Could you check a few things on this model? Use its own coordinates, in mm. A direction names the side the tool comes from. Coordinates: 2 decimals unless noted, no trailing zeros. Order: outer loops, then holes, each group sorted by start corner. A loop starts at its lowest first (then second) coordinate and runs counter-clockwise, first axis right, second up. Notation, with made-up numbers: (74, -20.5) - (85, -20.5) arc R18 ccw to (85, -9.5) - close; hole circle Ø6 at (38, 7.25). An arc over 180 degrees is marked (long way). One line per item, written item: value.
Autodesk Inventor part; units mm, degrees
ref_plane "Work Plane1" through (18.7433, 3, 13) normal (0, -1, 0) x (1, 0, 0)
ref_plane "YZ Plane" through (0, 0, 0) normal (1, 0, 0) x (0, 1, 0)
ref_plane "XZ Plane" through (0, 0, 0) normal (0, 1, 0) x (-1, 0, 0)
sketch "Sketch1" plane through (0, 0, 0) normal (0, 0, 1) x (1, 0, 0)
  circle A0 centre (0, 0) radius 38.75
  line L0 (-0.5, 39) -> (0.5, 39)
  line L1 (0.5, 39) -> (0.5, 31)
  line L2 (0.5, 31) -> (-0.5, 31)
  line L3 (-0.5, 31) -> (-0.5, 39)
  line L4 (-15.933, 26.5968) -> (-19.933, 33.525)
  line L5 (-19.067, 34.025) -> (-15.067, 27.0968)
  line L6 (-15.067, 27.0968) -> (-15.933, 26.5968)
  line L7 (-19.933, 33.525) -> (-19.067, 34.025)
  line L8 (-27.0968, 15.067) -> (-34.025, 19.067)
  line L9 (-33.525, 19.933) -> (-26.5968, 15.933)
  line L10 (-26.5968, 15.933) -> (-27.0968, 15.067)
  line L11 (-34.025, 19.067) -> (-33.525, 19.933)
  line L12 (-31, -0.5) -> (-39, -0.5)
  line L13 (-39, 0.5) -> (-31, 0.5)
  line L14 (-31, 0.5) -> (-31, -0.5)
  line L15 (-39, -0.5) -> (-39, 0.5)
  line L16 (-26.5968, -15.933) -> (-33.525, -19.933)
  line L17 (-34.025, -19.067) -> (-27.0968, -15.067)
  line L18 (-27.0968, -15.067) -> (-26.5968, -15.933)
  line L19 (-33.525, -19.933) -> (-34.025, -19.067)
  line L20 (-15.067, -27.0968) -> (-19.067, -34.025)
  line L21 (-19.933, -33.525) -> (-15.933, -26.5968)
  line L22 (-15.933, -26.5968) -> (-15.067, -27.0968)
  line L23 (-19.067, -34.025) -> (-19.933, -33.525)
  line L24 (0.5, -31) -> (0.5, -39)
  line L25 (-0.5, -39) -> (-0.5, -31)
  line L26 (-0.5, -31) -> (0.5, -31)
  line L27 (0.5, -39) -> (-0.5, -39)
  line L28 (15.933, -26.5968) -> (19.933, -33.525)
  line L29 (19.067, -34.025) -> (15.067, -27.0968)
  line L30 (15.067, -27.0968) -> (15.933, -26.5968)
  line L31 (19.933, -33.525) -> (19.067, -34.025)
  line L32 (27.0968, -15.067) -> (34.025, -19.067)
  line L33 (33.525, -19.933) -> (26.5968, -15.933)
  line L34 (26.5968, -15.933) -> (27.0968, -15.067)
  line L35 (34.025, -19.067) -> (33.525, -19.933)
  line L36 (31, 0.5) -> (39, 0.5)
  line L37 (39, -0.5) -> (31, -0.5)
  line L38 (31, -0.5) -> (31, 0.5)
  line L39 (39, 0.5) -> (39, -0.5)
  line L40 (26.5968, 15.933) -> (33.525, 19.933)
  line L41 (34.025, 19.067) -> (27.0968, 15.067)
  line L42 (27.0968, 15.067) -> (26.5968, 15.933)
  line L43 (33.525, 19.933) -> (34.025, 19.067)
  line L44 (15.067, 27.0968) -> (19.067, 34.025)
  line L45 (19.933, 33.525) -> (15.933, 26.5968)
  line L46 (15.933, 26.5968) -> (15.067, 27.0968)
  line L47 (19.067, 34.025) -> (19.933, 33.525)
  point P0 (0, 31)
  point P1 (-0.5, 38.7468)
  point P2 (0.5, 38.7468)
  point P3 (-15.5, 26.8468)
  point P4 (-26.8468, 15.5)
  point P5 (-31, 0)
  point P6 (-26.8468, -15.5)
  point P7 (-15.5, -26.8468)
  point P8 (0, -31)
  point P9 (15.5, -26.8468)
  point P10 (26.8468, -15.5)
  point P11 (31, 0)
  point P12 (26.8468, 15.5)
  point P13 (15.5, 26.8468)
  point P14 (-18.9404, 33.8057)
  point P15 (-19.8064, 33.3057)
  point P16 (-33.3057, 19.8064)
  point P17 (-33.8057, 18.9404)
  point P18 (-38.7468, 0.5)
  point P19 (-38.7468, -0.5)
  point P20 (-33.8057, -18.9404)
  point P21 (-33.3057, -19.8064)
  point P22 (-19.8064, -33.3057)
  point P23 (-18.9404, -33.8057)
  point P24 (-0.5, -38.7468)
  point P25 (0.5, -38.7468)
  point P26 (18.9404, -33.8057)
  point P27 (19.8064, -33.3057)
  point P28 (33.3057, -19.8064)
  point P29 (33.8057, -18.9404)
  point P30 (38.7468, -0.5)
  point P31 (38.7468, 0.5)
  point P32 (33.8057, 18.9404)
  point P33 (33.3057, 19.8064)
  point P34 (19.8064, 33.3057)
  point P35 (18.9404, 33.8057)
  dimension "d0" = 77.5
  dimension "d3" = 0.5
  dimension "d4" = 31
  dimension "d9" = 360
extrude "Extrusion1" add sketch "Sketch1" along normal blind 3 contours L36 L38 L37 A0 L32 L34 L33 L28 L30 L29 L24 L26 L25 L20 L22 L21 L16 L18 L17 L12 L14 L13 L8 L10 L9 L4 L6 L5 L3 L2 L1 L44 L46 L45 L40 L42 L41 | L41 L42 L40 A0 | A0 L40 L43 L41 | L32 L35 L33 A0 | A0 L33 L34 L32 | L1 L2 L3 A0 | A0 L3 L0 L1 | L24 L27 L25 A0 | A0 L25 L26 L24 | L9 L10 L8 A0 | A0 L8 L11 L9 | L16 L19 L17 A0 | A0 L17 L18 L16
sketch "Sketch2" plane through (0, 0, 3) normal (0, 0, 1) x (1, 0, 0)
  circle A0 centre (0, 0) radius 18.75
  circle A1 centre (0, 0) radius 26
  dimension "d11" = 37.5
  dimension "d12" = 52
extrude "Extrusion2" add sketch "Sketch2" along normal blind 10
sketch "Sketch3" plane through (0, 0, 3) normal (0, 0, 1) x (1, 0, 0)
  circle A0 centre (0, 0) radius 18.75
extrude "Extrusion3" cut sketch "Sketch3" against normal blind 10
sketch "Sketch4" plane through (0, 0, 13) normal (0, 0, 1) x (1, 0, 0)
  arc A0 (33.8057, -18.9404) -> (38.7468, -0.5) centre (0, 0) ccw
  line L0 (38.7468, -0.5) -> (17.4484, -0.5)
  line L1 (17.4484, -0.5) -> (17.4484, 0.5)
  line L2 (17.4484, 0.5) -> (38.7468, 0.5)
  line L3 (38.7468, 0.5) -> (38.7468, -0.5)
  line L4 (31, 1) -> (40.0251, 1)
  line L5 (40.0251, 1) -> (40.0251, -1)
  line L6 (40.0251, -1) -> (31, -1)
  line L7 (31, -1) -> (31, 1)
  point P0 (31, -0.5)
  point P1 (31, 0.5)
  dimension "d19" = 2
  dimension "d20" = 0.5
extrude "Extrusion4" cut sketch "Sketch4" against normal through all
sketch "Sketch5" plane through (18.7433, 0.5, 13) normal (0, -1, 0) x (1, 0, 0)
  circle A0 centre (3.7, -5) radius 1.6
  line L0 (14.5624, -10) -> (1.0631, -10)
  line L1 (-37.4933, 0) -> (0, 0)
  line L2 (0, 0) -> (0, -10)
  point P0 (-18.7433, -13)
  point P1 (0, -5)
  dimension "d21" = 3.2
  dimension "d22" = 5
  dimension "d23" = 3.7
extrude "Extrusion5" cut sketch "Sketch5" against normal blind 23.5
ref_plane "Work Plane1" through (18.7433, 3, 13) normal (0, -1, 0) x (1, 0, 0)
sketch "Sketch6" plane through (18.7433, 3, 13) normal (0, -1, 0) x (1, 0, 0)
  circle A0 centre (3.7, -5) radius 1.6
  circle A1 centre (3.7, -5) radius 3.25
  point P0 (-18.7433, -13)
  dimension "d27" = 6.5
extrude "Extrusion6" cut sketch "Sketch6" against normal blind 23.5
mirror "Mirror1" about plane through (0, 0, 0) normal (0, 1, 0) of "Extrusion6", "Extrusion5"
chamfer "Chamfer1" distance 1 angle 45 2 edges at (-18.75, 0, 13) (-18.75, 0, 0)
sketch "Sketch7" plane through (0, 0, 3) normal (0, 0, 1) x (1, 0, 0)
  circle A0 centre (0, 0) radius 38.75
  arc A1 (18.9404, 33.8057) -> (0.5, 38.7468) centre (0, 0) ccw
  circle A2 centre (0, 0) radius 41.405
extrude "Extrusion7" cut sketch "Sketch7" against normal blind 3
properties part number "disk_6_slot"
Item 1: I want a section at B-B on z = 8. Please give me the cut outline in (x, y), then the cut area to 3 significant figures.
Conclusion:
outline: (18.74, -0.5) arc R18.75 cw (long way) to (18.74, 0.5) - (20.84, 0.5) - (20.84, 3) - (19.19, 3) - (19.19, 17.54) arc R26 ccw (long way) to (19.19, -17.54) - (19.19, -3) - (20.84, -3) - (20.84, -0.5) - close; (24.04, -3) - (25.69, -3) - (25.69, -3.98) arc R26 ccw to (26, -0.5) - (24.04, -0.5) - close; (24.04, 0.5) - (26, 0.5) arc R26 ccw to (25.69, 3.98) - (25.69, 3) - (24.04, 3) - close
area: 873 mm²
Item 2: I'm going to push flat-ended pins straight in: pin 1 Ø0.8 at (y, z) = (0, 1.5) entering from -X; pin 2 Ø6 at (x, z) = (-31, 1.5) entering from +Y; pin 3 Ø2 at (y, z) = (-13.5, 9.5) entering from -X; pin 4 Ø8 at (x, y) = (-18.5, -15.5) entering from -Z. Where does each tip first touch, or does it pass through?
Conclusion:
pin 1: x = -31
pin 2: y = 26.79
pin 3: x = -22.8
pin 4: z = 0
Item 3: I want a section at C-C on y = 32. Please give me the cut outline in (x, z).
Conclusion:
outline: (-21.85, 0) - (-19.05, 0) - (-19.05, 3) - (-21.85, 3) - close; (-17.9, 0) - (17.9, 0) - (17.9, 3) - (-17.9, 3) - close; (19.05, 0) - (21.85, 0) - (21.85, 3) - (19.05, 3) - close
Item 4: For faces 4 (the face through (35, -1, 2)), 5 (the face through (19.196, 8.553, 8.143)), 6 (the face through (-35, -0.5, 1)), which set-ups out of +Z, -Z, +X, -X, +Y, -Y let a thin tool reach every point of the face, with its end or its side?
Conclusion:
face 4: +Z, -Z, +X
face 5: +Y
face 6: +Z, -Z, -X
Item 5: If I drill on probe 1 along Y at (x, z) = (0, 4.5); probe 2 along X at (y, z) = (-8.5, 8); probe 3 along Z at (x, y) = (-2.5, -29.5), over which ranges is the centre line in solid material (lowest first)?
Conclusion:
probe 1: -26 to -18.75, 18.75 to 26
probe 2: -24.57 to -16.71, 16.71 to 19.19
probe 3: 0 to 3
Item 6: I want a section at A-A on x = 0. Please give me the cut outline in (y, z).
Conclusion:
outline: (-38.75, 0) - (-19.75, 0) - (-18.75, 1) - (-18.75, 12) - (-19.75, 13) - (-26, 13) - (-26, 3) - (-38.75, 3) - close; (18.75, 1) - (19.75, 0) - (38.75, 0) - (38.75, 3) - (26, 3) - (26, 13) - (19.75, 13) - (18.75, 12) - close
Item 7: I want a section at D-D on x = -28.5. Please give me the cut outline in (y, z), then the cut area to 3 significant figures.
Conclusion:
outline: (-26.25, 0) - (26.25, 0) - (26.25, 3) - (-26.25, 3) - close
area: 158 mm²
Item 8: Thinking about a two-plate mould opening in Y: for faces 1 (the face through (21.17, -1.73, 8.97)), 2 (the face through (-25.975, -1.136, 7.93)), 3 (the face through (23, 0.5, 5)), which applies, pulls with the +Y half, pulls with the -Y half, needs draft (parallel to the pull), parting line crosses it, or undercut?
Conclusion:
face 1: needs draft
face 2: parting line crosses it
face 3: undercut
